Geometry: final body of the model. Coordinates: model frame, mm. A direction names the side the tool comes from. Give positions to 0.01 mm unless a question says otherwise; leave off trailing zeros. Loops run counter-clockwise (first coordinate to the right, second up) from the corner with the lowest first, then second, coordinate; pieces in that order, holes last.
from build123d import *

# Parameters (mm, degrees)
F1_R     = 2.578
F1_W     = 24
F1_H     = 4
F2_DEPTH = 3.175
F3_R     = 2
F4_R     = 1


# Not quite as in the source:
# - a feature names something its author has since deleted; it is built from what else it names


with BuildPart() as f2:
    # F1 (on Front) → F2 (new body)
    with BuildSketch(Plane.XZ):
        Polygon((45.5, 49.5), (45.5, 80.5), (-45.5, 80.5), (-45.5, -80.5), (-5, -80.5), (-5, -77), (5, -77), (5, -80.5), (45.5, -80.5), (45.5, -0.5), (39, -0.5), (39, 49.5), align=None)
        with Locations((-41.4446451293, -76.6580848593)):
            Circle(F1_R, mode=Mode.SUBTRACT)
        with Locations((0, -60.5)):
            Rectangle(F1_W, F1_H, mode=Mode.SUBTRACT)
        with Locations((41.4446451293, -76.6580848593)):
            Circle(F1_R, mode=Mode.SUBTRACT)
        with Locations((-41.4446451293, 76.6580848593)):
            Circle(F1_R, mode=Mode.SUBTRACT)
        with BuildLine():
            ThreePointArc((-7.5, 58), (0, 65.5), (7.5, 58))
            Line((7.5, 58), (7.5, 25))
            ThreePointArc((7.5, 25), (0, 17.5), (-7.5, 25))
            Line((-7.5, 25), (-7.5, 58))
        make_face(mode=Mode.SUBTRACT)
        with Locations((41.4446451293, 76.6580848593)):
            Circle(F1_R, mode=Mode.SUBTRACT)
    extrude(amount=F2_DEPTH)

    # F3
    f3_edges = [f2.edges().sort_by_distance(p)[0] for p in [
        (-45.5, -1.5875, 80.5),
        (45.5, -1.5875, 80.5),
        (45.5, -1.5875, 49.5),
        (39, -1.5875, 49.5),
        (45.5, -1.5875, -0.5),
        (39, -1.5875, -0.5),
        (-45.5, -1.5875, -80.5),
        (45.5, -1.5875, -80.5),
    ]]
    fillet(f3_edges, radius=F3_R)

    # F4
    f4_edges = [f2.edges().sort_by_distance(p)[0] for p in [
        (5, -1.5875, -80.5),
        (5, -1.5875, -77),
        (-5, -1.5875, -77),
        (-5, -1.5875, -80.5),
    ]]
    fillet(f4_edges, radius=F4_R)


solid = f2.part
Item 1: Section query A-A on x = 0. Return loops of the section in (y, z) (3 decimals).
Values follow:
outline: (-3.175, -77) - (0, -77) - (0, -62.5) - (-3.175, -62.5) - close; (-3.175, -58.5) - (0, -58.5) - (0, 17.5) - (-3.175, 17.5) - close; (-3.175, 65.5) - (0, 65.5) - (0, 80.5) - (-3.175, 80.5) - close
Item 2: Set-up query: faces 5 (the face through (39, -2, 24)), 6 (the face through (0, -2, -77)), 7 (the face through (0, -2, -58.5)). Return all of +Z, -Z, +X, -X, +Y, -Y with unobstructed straight access to the full face (end or side cutting, diameter ignored); none if empty.
Values follow:
face 5: +X, +Y, -Y
face 6: -Z, +Y, -Y
face 7: +Y, -Y
Item 3: Ray query, probe 1 along Z at (x, y) = (-1, -2.35); probe 2 along Z at (x, y) = (6, -2.7); probe 3 along X at (y, z) = (-2.8, 36). Return the intervals inside material, ascending.
Values follow:
probe 1: z = -77 to -62.5, -58.5 to 17.57, 65.43 to 80.5
probe 2: z = -80.5 to -62.5, -58.5 to 20.5, 62.5 to 80.5
probe 3: x = -45.5 to -7.5, 7.5 to 39
Item 4: Section query B-B on z = 5. Return loops of the section in (x, y) (3 decimals).
Values follow:
outline: (-45.5, -3.175) - (39, -3.175) - (39, 0) - (-45.5, 0) - close
Item 5: Draft query along X for faces 1 (the face through (1, -2, 80.5)), 2 (the face through (40.89, -1.57, 74.14)), 3 (the face through (0, -2, -62.5)), 4 (the face through (45.5, -2, -41)). Return one class per face: +X half, -X half, draft (parallel to the pull), parting line (faces both ways), or undercut.
Values follow:
face 1: draft
face 2: undercut
face 3: undercut
face 4: +X half
Item 6: Pin query (flat end, axial travel): pin 1 (8 mm diameter, centred on x = 41.44, z = -76.66, fed in from +Y); pin 2 (4 mm diameter, centred on x = -41.44, z = 76.66, fed in from -Y). Return the tip coordinate at first contact, or that it passes through.
Values follow:
pin 1: stops at y = 0
pin 2: passes through
